```python
from build123d import *

# Parameters (mm, degrees)
BOSS_EXTRUDE1_DEPTH      = 3
BOSS_EXTRUDE1_DEPTH_BACK = 7


with BuildPart() as part:
    # Sketch1 → Boss-Extrude1 (new, two sides: drawn at the far end of the back side and taken through both)
    with BuildSketch(Plane(origin=(0, 0, 0), x_dir=(1, 0, 0), z_dir=(0, 1, 0)).offset(-BOSS_EXTRUDE1_DEPTH_BACK)):
        Polygon((-5.773502692, -10), (5.773502692, -10), (11.547005384, 0), (5.773502692, 10), (-5.773502692, 10), (-11.547005384, 0), align=None)
    extrude(amount=BOSS_EXTRUDE1_DEPTH + BOSS_EXTRUDE1_DEPTH_BACK)


solid = part.part
```
The listing builds one solid part. Answer for the finished solid, in the listing's coordinates (mm). Give positions to 0.01 mm unless a question says otherwise; leave off trailing zeros. Order: outer loops, then holes, each group sorted by start corner. A loop starts at its lowest first (then second) coordinate and runs counter-clockwise, first axis right, second up. Notation, with made-up numbers: (9, 47) -> (16, 47) arc R24 ccw to (16, 60) -> close; hole circle Ø11 at (-36, 80.25). An arc over 180 degrees is marked (long way). One line per item, written item: value.
1) A flat-ended cylindrical pin translates along its axis: P1, Ø3, axis at y = -4.5, z = 3, coming from the +X side. Find the tip coordinate at first contact, or state that the pin passes through.
Reported:
P1: stops at x = 10.68
2) Find section A-A, the plane y = -1.5. Determine the outline of the cut face in (x, z).
Reported:
outline: (-11.55, 0) -> (-5.77, -10) -> (5.77, -10) -> (11.55, 0) -> (5.77, 10) -> (-5.77, 10) -> close
3) Find the intervals of material crossed by line 1 (X direction, y = -3, z = -3); line 2 (Z direction, x = -6, y = 0.75); line 3 (X direction, y = -0.5, z = 1.25), in increasing order.
Reported:
line 1: x = -9.81 to 9.81
line 2: z = -9.61 to 9.61
line 3: x = -10.83 to 10.83
4) Find section B-B, the plane x = 8.5. Determine the outline of the cut face in (y, z), plus the area to 3 significant figures.
Reported:
outline: (-7, -5.28) -> (3, -5.28) -> (3, 5.28) -> (-7, 5.28) -> close
area: 106 mm^2
5) Find section C-C, the plane z = 7.75. Determine the outline of the cut face in (x, y).
Reported:
outline: (-7.07, -7) -> (7.07, -7) -> (7.07, 3) -> (-7.07, 3) -> close
